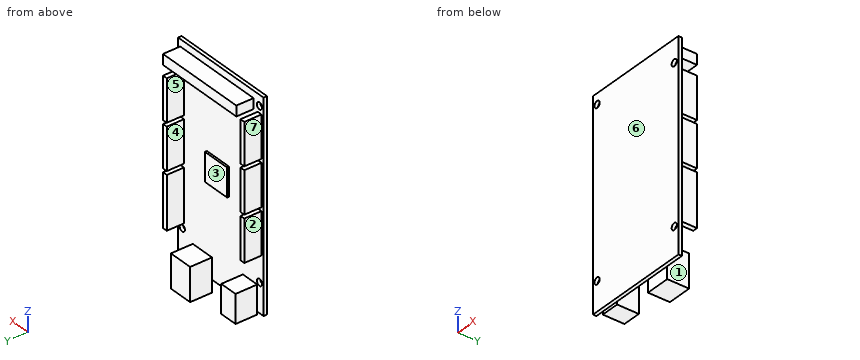
Autodesk Inventor part; units mm, degrees
ref_plane "YZ Plane" through (0, 0, 0) normal (1, 0, 0) x (0, 1, 0)
ref_plane "XZ Plane" through (0, 0, 0) normal (0, 1, 0) x (-1, 0, 0)
ref_plane "XY Plane" through (0, 0, 0) normal (0, 0, 1) x (1, 0, 0)
sketch "Sketch1" plane through (0, 0, 0) normal (0, 1, 0) x (-1, 0, 0)
  line L0 (-26.85, 50.85) -> (26.85, 50.85)
  line L1 (26.85, 50.85) -> (26.85, -50.85)
  line L2 (26.85, -50.85) -> (-26.85, -50.85)
  line L3 (-26.85, -50.85) -> (-26.85, 50.85)
  line L4 (-26.85, 50.85) -> (26.85, -50.85) construction
  line L5 (26.85, 50.85) -> (-26.85, -50.85) construction
  point P0 (0, 0)
  dimension "d0" = 53.7
  dimension "d1" = 101.7
extrude "Extrusion1" add sketch "Sketch1" along normal blind 1.7
sketch "Sketch2" plane through (0, 1.7, 0) normal (0, 1, 0) x (1, 0, 0)
  line L0 (26.85, 50.85) -> (-26.85, 50.85)
  line L1 (-26.85, 50.85) -> (-26.85, -50.85)
  line L2 (-22.85, 38.25) -> (-13.85, 38.25)
  line L3 (-13.85, 38.25) -> (-13.85, 52.25)
  line L4 (-13.85, 52.25) -> (-22.85, 52.25)
  line L5 (-22.85, 52.25) -> (-22.85, 38.25)
  point P0 (0, 0)
  dimension "d6" = 9
  dimension "d7" = 14
extrude "Extrusion2" add sketch "Sketch2" along normal blind 10.7
sketch "Sketch3" plane through (0, 1.7, 0) normal (0, 1, 0) x (1, 0, 0)
  line L0 (26.85, 50.85) -> (-26.85, 50.85)
  line L1 (17.65, 40.45) -> (5.55, 40.45)
  line L2 (5.55, 40.45) -> (5.55, 56.85)
  line L3 (5.55, 56.85) -> (17.65, 56.85)
  line L4 (17.65, 56.85) -> (17.65, 40.45)
  point P0 (0, 0)
  dimension "d12" = 12.1
  dimension "d13" = 16.4
extrude "Extrusion3" add sketch "Sketch3" along normal blind 10.8
sketch "Sketch4" plane through (0, 1.7, 0) normal (0, 1, 0) x (1, 0, 0)
  line L0 (-26.85, -50.85) -> (26.85, -50.85)
  line L1 (-26.85, 50.85) -> (-26.85, -50.85)
  line L2 (-20.55, -47.35) -> (25.55, -47.35)
  line L3 (25.55, -47.35) -> (25.55, -42.25)
  line L4 (25.55, -42.25) -> (-20.55, -42.25)
  line L5 (-20.55, -42.25) -> (-20.55, -47.35)
  point P0 (0, 0)
  dimension "d18" = 46.1
  dimension "d19" = 5.1
extrude "Extrusion4" add sketch "Sketch4" along normal blind 8.5
sketch "Sketch5" plane through (0, 1.7, 0) normal (0, 1, 0) x (1, 0, 0)
  line L0 (-26.85, -50.85) -> (26.85, -50.85)
  line L1 (-25.55, -42.35) -> (-23.15, -42.35)
  line L2 (-23.15, -42.35) -> (-23.15, -21.65)
  line L3 (-23.15, -21.65) -> (-25.55, -21.65)
  line L4 (-25.55, -21.65) -> (-25.55, -42.35)
  line L5 (-25.55, -19.85) -> (-23.15, -19.85)
  line L6 (-23.15, -19.85) -> (-23.15, 0.85)
  line L7 (-23.15, 0.85) -> (-25.55, 0.85)
  line L8 (-25.55, 0.85) -> (-25.55, -19.85)
  line L9 (-25.55, 2.65) -> (-23.15, 2.65)
  line L10 (-23.15, 2.65) -> (-23.15, 23.35)
  line L11 (-23.15, 23.35) -> (-25.55, 23.35)
  line L12 (-25.55, 23.35) -> (-25.55, 2.65)
  line L13 (25.55, -37.25) -> (23.15, -37.25)
  line L14 (23.15, -37.25) -> (23.15, -16.55)
  line L15 (23.15, -16.55) -> (25.55, -16.55)
  line L16 (25.55, -16.55) -> (25.55, -37.25)
  line L17 (25.55, -14.75) -> (23.15, -14.75)
  line L18 (23.15, -14.75) -> (23.15, 5.95)
  line L19 (23.15, 5.95) -> (25.55, 5.95)
  line L20 (25.55, 5.95) -> (25.55, -14.75)
  line L21 (25.55, 7.75) -> (23.15, 7.75)
  line L22 (23.15, 7.75) -> (23.15, 33.75)
  line L23 (23.15, 33.75) -> (25.55, 33.75)
  line L24 (25.55, 33.75) -> (25.55, 7.75)
  point P0 (0, 0)
  dimension "d24" = 2.4
  dimension "d25" = 20.7
  dimension "d26" = 1.8
  dimension "d27" = 20.7
  dimension "d28" = 1.8
  dimension "d29" = 20.7
  dimension "d32" = 2.4
  dimension "d33" = 20.7
  dimension "d34" = 1.8
  dimension "d35" = 20.7
  dimension "d36" = 1.8
  dimension "d37" = 26
extrude "Extrusion5" add sketch "Sketch5" along normal blind 8.5
sketch "Sketch6" plane through (0, 1.7, 0) normal (0, 1, 0) x (1, 0, 0)
  line L0 (-22.85, 50.85) -> (-26.85, 50.85)
  line L1 (-26.85, 50.85) -> (-26.85, -50.85)
  line L2 (-5.25, 6.55) -> (8.75, 6.55)
  line L3 (8.75, 6.55) -> (8.75, -7.45)
  line L4 (8.75, -7.45) -> (-5.25, -7.45)
  line L5 (-5.25, -7.45) -> (-5.25, 6.55)
  point P0 (0, 0)
  dimension "d42" = 14
  dimension "d43" = 14
extrude "Extrusion6" add sketch "Sketch6" along normal blind 1
sketch "Sketch7" plane through (0, 1.7, 0) normal (0, 1, 0) x (1, 0, 0)
  circle A0 centre (-24.25, 36.5) radius 1.65
  point P0 (0, 0)
  point P1 (-26.85, 50.85)
  dimension "d48" = 3.3
  dimension "d64" = 14.35
extrude "Extrusion7" cut sketch "Sketch7" against normal blind 2
mirror "Mirror1" about plane through (0, 0, 0) normal (1, 0, 0) of "Extrusion7"
sketch "Sketch8" plane through (0, 1.7, 0) normal (0, 1, 0) x (1, 0, 0)
  line L0 (-26.85, -50.85) -> (26.85, -50.85)
  line L1 (-26.85, 50.85) -> (-26.85, -50.85)
  circle A0 centre (-24.25, -45.65) radius 1.65
  point P0 (0, 0)
  dimension "d53" = 3.3
  dimension "d63" = 96.5
extrude "Extrusion8" cut sketch "Sketch8" against normal blind 2
sketch "Sketch9" plane through (0, 1.7, 0) normal (0, 1, 0) x (1, 0, 0)
  line L0 (23.15, 5.95) -> (23.15, -14.75)
  circle A0 centre (24.25, -39.75) radius 1.65
  line L1 (23.15, -37.25) -> (25.55, -37.25)
  point P0 (0, 0)
  point P1 (26.85, 50.85)
  dimension "d59" = 3.3
  dimension "d60" = 2.5
extrude "Extrusion9" cut sketch "Sketch9" against normal blind 2
properties part number "ArduinoMega"
Read the model definition and answer for the solid it produces. Units are mm, in the model's axes. Face numbers are marked on the shaded views. A direction names the side the tool comes from. Round coordinates to 2 decimals unless told otherwise and drop trailing zeros. Write each loop counter-clockwise with the first axis right and the second up, starting at its lowest first coordinate (ties: lowest second). Pieces come first, ordered by that corner, then holes. Notation, with made-up numbers: (7, 5) -> (40, 5) arc R28 ccw to (40, 30) -> close; hole circle Ø3 at (-12.75, -3). An arc over 180 degrees is marked (long way). Answer in a Markdown table with one row per item. Add a question column.
1) Find section C-C, the plane z = -36.5. Determine the outline of the cut face in (x, y), and give its area (3 significant figures).
2) Which of the six approach directions +Z, -Z, +X, -X, +Y, -Y give full straight-line access (tool end or side, diameter ignored) to the marked faces 1, 2, 3 and 4?
3) Consider line 1 (Z direction, x = -24.25, y = 0.8); line 2 (Z direction, x = 24.25, y = 0.9); line 3 (Z direction, x = 24.5, y = 5.25). Determine where each line is inside the solid, lowest interval first.
4) Find section A-A, the plane x = 24.25. Determine the outline of the cut face in (y, z), and give its area (3 significant figures).
5) Determine the mould class of the marked faces 5, 6 and 7 for opening direction X: pulls with the +X half, pulls with the -X half, needs draft (parallel to the pull), parting line crosses it, or undercut.
6) Find section B-B, the plane z = 39.75. Determine the outline of the cut face in (x, y).
7) Given P1, Ø1.9, axis at x = -25, z = -10.5, coming from the +Y side; P2, Ø1.5, axis at x = 0.5, z = -30.5, coming from the +Y side; P3, Ø0.7, axis at x = 24.5, y = 6.5, coming from the -Z side, each flat-ended and moving along its own axis, determine where each tip first touches the part or whether it passes through.
8) Find section D-D, the plane x = 11. Determine the outline of the cut face in (y, z), and give its area (3 significant figures).
Findings below:
| question | item | result |
|---|---|---|
| 1 | outline | (-26.85, 0) -> (-25.9, 0) -> (-25.9, 1.7) -> (-26.85, 1.7) -> close; (-22.6, 0) -> (22.6, 0) -> (22.6, 1.7) -> (-22.6, 1.7) -> close; (25.9, 0) -> (26.85, 0) -> (26.85, 1.7) -> (25.9, 1.7) -> close |
| 1 | area | 80.1 mm² |
| 2 | face 1 | -Z, +X, +Y |
| 2 | face 2 | +Z, -Z, -X, +Y |
| 2 | face 3 | +Y |
| 2 | face 4 | -Z, +Y |
| 3 | line 1 | -50.85 to -38.15, -34.85 to 44, 47.3 to 50.85 |
| 3 | line 2 | -50.85 to -38.15, -34.85 to 38.1, 41.4 to 50.85 |
| 3 | line 3 | -33.75 to -7.75, -5.95 to 14.75, 16.55 to 37.25, 42.25 to 47.35 |
| 4 | outline | (0, -50.85) -> (1.7, -50.85) -> (1.7, -38.15) -> (0, -38.15) -> close; (0, -34.85) -> (1.7, -34.85) -> (1.7, -33.75) -> (10.2, -33.75) -> (10.2, -7.75) -> (1.7, -7.75) -> (1.7, -5.95) -> (10.2, -5.95) -> (10.2, 14.75) -> (1.7, 14.75) -> (1.7, 16.55) -> (10.2, 16.55) -> (10.2, 37.25) -> (1.7, 37.25) -> (1.7, 38.1) -> (0, 38.1) -> close; (0, 41.4) -> (1.7, 41.4) -> (1.7, 42.25) -> (10.2, 42.25) -> (10.2, 47.35) -> (1.7, 47.35) -> (1.7, 50.85) -> (0, 50.85) -> close |
| 4 | area | 778 mm² |
| 5 | face 5 | undercut |
| 5 | face 6 | needs draft |
| 5 | face 7 | pulls with the -X half |
| 6 | outline | (-26.85, 0) -> (22.6, 0) -> (22.6, 1.7) -> (-23.15, 1.7) -> (-23.15, 10.2) -> (-25.55, 10.2) -> (-25.55, 1.7) -> (-26.85, 1.7) -> close; (25.9, 0) -> (26.85, 0) -> (26.85, 1.7) -> (25.9, 1.7) -> close |
| 7 | P1 | y = 10.2 |
| 7 | P2 | y = 1.7 |
| 7 | P3 | z = -33.75 |
| 8 | outline | (0, -50.85) -> (1.7, -50.85) -> (1.7, -56.85) -> (12.5, -56.85) -> (12.5, -40.45) -> (1.7, -40.45) -> (1.7, 42.25) -> (10.2, 42.25) -> (10.2, 47.35) -> (1.7, 47.35) -> (1.7, 50.85) -> (0, 50.85) -> close |
| 8 | area | 393 mm² |
